Autodesk Inventor part; units mm, degrees
ref_plane "YZ Plane" through (0, 0, 0) normal (1, 0, 0) x (0, 1, 0)
ref_plane "XZ Plane" through (0, 0, 0) normal (0, 1, 0) x (-1, 0, 0)
ref_plane "XY Plane" through (0, 0, 0) normal (0, 0, 1) x (1, 0, 0)
sketch "Sketch2" plane through (0, 0, 0) normal (0, 0, 1) x (1, 0, 0)
  line L0 (-20.195, -14.5) -> (20.195, -14.5)
  line L1 (20.195, -14.5) -> (20.195, 14.5)
  line L2 (20.195, 14.5) -> (-20.195, 14.5)
  line L3 (-20.195, 14.5) -> (-20.195, -14.5)
  line L4 (-20.195, -14.5) -> (20.195, 14.5) construction
  line L5 (20.195, -14.5) -> (-20.195, 14.5) construction
  point P0 (0, 0)
  dimension "d0" = 40.39
  dimension "d1" = 29
extrude "Extrusion1" add sketch "Sketch2" along normal blind 18.75
sketch "Sketch3" plane through (-20.195, 14.5, 0) normal (0, 1, 0) x (1, 0, 0)
  line L0 (40.39, 0) -> (0, 0) construction
  line L1 (0, 0) -> (0, -18.75) construction
  line L2 (40.39, -18.75) -> (0, -18.75) construction
  line L3 (40.39, 0) -> (40.39, -18.75) construction
  line L4 (0, 0) -> (40.39, -18.75) construction
  line L5 (-7.045, -18.75) -> (47.435, -18.75)
  line L6 (47.435, -18.75) -> (47.435, 0)
  line L7 (47.435, 0) -> (-7.045, 0)
  line L8 (-7.045, 0) -> (-7.045, -18.75)
  line L9 (-7.045, -18.75) -> (47.435, 0) construction
  line L10 (47.435, -18.75) -> (-7.045, 0) construction
  line L11 (-7.045, -9.375) -> (47.435, -9.375) construction
  circle A0 centre (-4.75, -4.15) radius 2.1
  line L12 (20.195, -9.375) -> (20.195, -3.4775) construction
  circle A1 centre (-4.75, -14.6) radius 2.1
  circle A2 centre (45.14, -4.15) radius 2.1
  circle A3 centre (45.14, -14.6) radius 2.1
  point P0 (20.195, 0)
  dimension "d4" = 54.48
  dimension "d5" = 4.2
  dimension "d6" = 4.15
  dimension "d7" = 4.75
extrude "Extrusion2" add sketch "Sketch3" along normal blind 2.22
sketch "Sketch4" plane through (-20.195, 16.72, 0) normal (0, 1, 0) x (1, 0, 0)
  line L0 (0, 0) -> (0, -18.75)
  line L1 (40.39, 0) -> (40.39, -18.75)
  line L2 (47.435, 0) -> (-7.045, 0)
  line L3 (-7.045, -18.75) -> (47.435, -18.75)
  point P0 (20.195, 0)
extrude "Extrusion3" add sketch "Sketch4" along normal blind 9.42
sketch "Sketch5" plane through (-20.195, 26.14, 0) normal (0, 1, 0) x (1, 0, 0)
  line L0 (40.39, -18.75) -> (40.39, 0)
  line L1 (40.39, 0) -> (0, 0)
  line L2 (0, 0) -> (0, -18.75)
  line L3 (0, -18.75) -> (40.39, -18.75)
  line L4 (40.39, -9.375) -> (0, -9.375) construction
  circle A0 centre (30, -9.375) radius 2.865
  point P0 (20.195, 0)
  dimension "d12" = 30
  dimension "d13" = 5.73
extrude "Extrusion4" add sketch "Sketch5" along normal blind 5.77 contours A0
ref_plane "Work Plane1" through (0, 0, 9.375) normal (0, 0, 1) x (1, 0, 0)
properties part number "40kgServo"
Geometry check sheet. Reference: the model listing, model coordinates, mm. A direction names the side the tool comes from. Round coordinates to 2 decimals unless told otherwise and drop trailing zeros. Loops run counter-clockwise (first coordinate to the right, second up) from the corner with the lowest first, then second, coordinate; pieces in that order, holes last. Notation, with made-up numbers: (19.25, 7) -> (42.25, 7) arc R34 ccw to (42.25, 38) -> close; hole circle Ø9 at (-38.5, 40). An arc over 180 degrees is marked (long way). Use a Markdown table: item, result.
(1) Sectioned sample at A-A (z = 4.15). Enter the section's corners in (x, y) (3 decimals), then the cut area to 3 significant figures.
Calculated:
| item | result |
|---|---|
| outline | (-27.24, 14.5) -> (-27.045, 14.5) -> (-27.045, 16.72) -> (-27.24, 16.72) -> close; (-22.845, 14.5) -> (-20.195, 14.5) -> (-20.195, -14.5) -> (20.195, -14.5) -> (20.195, 14.5) -> (22.845, 14.5) -> (22.845, 16.72) -> (20.195, 16.72) -> (20.195, 26.14) -> (-20.195, 26.14) -> (-20.195, 16.72) -> (-22.845, 16.72) -> close; (27.045, 14.5) -> (27.24, 14.5) -> (27.24, 16.72) -> (27.045, 16.72) -> close |
| area | 1,650 mm² |
(2) Sectioned sample at D-D (x = -17.5). Enter the section's corners in (y, z), then the cut area to 3 significant figures.
Calculated:
| item | result |
|---|---|
| outline | (-14.5, 0) -> (26.14, 0) -> (26.14, 18.75) -> (-14.5, 18.75) -> close |
| area | 762 mm² |
(3) Scan lines: probe 1 along X at (y, z) = (15.7, 4.15) (3 decimals); probe 2 along X at (y, z) = (16.5, 3.25); probe 3 along Y at (x, z) = (23, 13.5). Record each from-to range of solid material in increasing order.
Calculated:
| item | result |
|---|---|
| probe 1 | -27.24 to -27.045, -22.845 to 22.845, 27.045 to 27.24 |
| probe 2 | -27.24 to -26.84, -23.05 to 23.05, 26.84 to 27.24 |
| probe 3 | 14.5 to 16.72 |
(4) Sectioned sample at B-B (y = 9.5). Enter the section's corners in (x, z) (3 decimals), then the cut area to 3 significant figures.
Calculated:
| item | result |
|---|---|
| outline | (-20.195, 0) -> (20.195, 0) -> (20.195, 18.75) -> (-20.195, 18.75) -> close |
| area | 757 mm² |
(5) Mould release check, pull along X, two halves, no side actions. Record for faces 6 (the flat face through (-27.24, 16, 9)), 7 (the flat face through (27.24, 16, 10)), 8 (the flat face through (0, 6, 18.75)), 9 (the cylindrical face through (-22.94, 15.59, 15.23)): released by +X, released by -X, zero draft, split by the parting line, or undercut.
Calculated:
| item | result |
|---|---|
| face 6 | released by -X |
| face 7 | released by +X |
| face 8 | zero draft |
| face 9 | undercut |
(6) Go/stop test with flat-tipped pins: P1, Ø5.5, axis at x = 23.5, z = 11.5, coming from the +Y side; P2, Ø5.5, axis at x = 24.945, z = 4.15, coming from the -Y side; P3, Ø1, axis at y = 4.5, z = 10.5, coming from the +X side (3 decimals). Record where each tip stops, or that it passes through.
Calculated:
| item | result |
|---|---|
| P1 | y = 16.72 |
| P2 | y = 14.5 |
| P3 | x = 20.195 |
(7) Set-up check for faces 1 (the flat face through (23, 14.5, 9)), 2 (the flat face through (-20.195, 21, 9)), 3 (the flat face through (-20.195, 0, 9)), 4 (the flat face through (20.195, 21, 9)), 5 (the cylindrical face through (11.35, 28.98, 11.79)): record each of +Z, -Z, +X, -X, +Y, -Y from which the full face is reachable in a straight line by a thin tool's end or side.
Calculated:
| item | result |
|---|---|
| face 1 | +Z, -Z, +X, -Y |
| face 2 | +Z, -Z, -X, +Y |
| face 3 | +Z, -Z, -X, -Y |
| face 4 | +Z, -Z, +X, +Y |
| face 5 | +Y |
(8) Sectioned sample at C-C (z = 10.5). Enter the section's corners in (x, y) (3 decimals).
Calculated:
| item | result |
|---|---|
| outline | (-27.24, 14.5) -> (-20.195, 14.5) -> (-20.195, -14.5) -> (20.195, -14.5) -> (20.195, 14.5) -> (27.24, 14.5) -> (27.24, 16.72) -> (20.195, 16.72) -> (20.195, 26.14) -> (12.44, 26.14) -> (12.44, 31.91) -> (7.17, 31.91) -> (7.17, 26.14) -> (-20.195, 26.14) -> (-20.195, 16.72) -> (-27.24, 16.72) -> close |
